```python
from build123d import *

# Parameters (mm, degrees)
SKETCH1_R           = 44.45
BOSS_EXTRUDE1_DEPTH = 1000


with BuildPart() as part:
    # Sketch1 → Boss-Extrude1 (new body)
    with BuildSketch(Plane(origin=(0, 0, 0), x_dir=(1, 0, 0), z_dir=(0, 1, 0))):
        with Locations(Location((0, 0, 0), (0, 0, 270))):
            Circle(SKETCH1_R)
    extrude(amount=BOSS_EXTRUDE1_DEPTH)

    # Sketch3 → Revolve3 (revolve)
    with BuildSketch(Plane.XY, mode=Mode.PRIVATE) as revolve3_sk:
        Polygon((0, 1000), (0, 1276.86), (-44.45, 1000), align=None)
    revolve(revolve3_sk.sketch.rotate(Axis((0, 1000, 0), (0, 1, 0)), 270), axis=Axis((0, 1000, 0), (0, 1, 0)))

    # Sketch4 → Revolve4 (revolve)
    with BuildSketch(Plane.XY):
        Polygon((0, 0), (0, -276.86), (-44.45, 0), align=None)
    revolve(axis=Axis((0, 0, 0), (0, -1, 0)))


solid = part.part
```
Here's how the part is built. I have some questions about the finished solid (model axes, mm). Coordinates: 2 decimals unless noted, no trailing zeros. Write each loop counter-clockwise with the first axis right and the second up, starting at its lowest first coordinate (ties: lowest second). Pieces come first, ordered by that corner, then holes. Notation, with made-up numbers: M 2.25,67 L 21.25,67 A24 cw 21.25,81 Z; hole C 73.25,-1 d1. An arc over 180 degrees is marked long. Answer as CSV lines item,"result". Start each with the question number.
Q1. Will these pins go through, and if not, where does the flat tip stop? pin 1 Ø1 at (y, z) = (57.5, -31.5) entering from -X; pin 2 Ø6 at (x, y) = (-3, 753.5) entering from -Z; pin 3 Ø1 at (y, z) = (978.5, 9) entering from -X; pin 4 Ø3 at (x, y) = (-5.5, 353.5) entering from +Z.
Q2. I need wall thicknesses on probe 1 along X at (y, z) = (796, -0.5); probe 2 along Z at (x, y) = (-22, 754); probe 3 along Z at (x, y) = (25, -33). Which ranges of each line are inside material? Lowest first, please. Write a range as [from, to].
Q3. Suppose I cut it at B-B, the plane y = -157. List the corners of the cut face in (x, z) for me, then the cut area to 3 significant figures.
Q4. Suppose I cut it at A-A, the plane y = 699. List the corners of the cut face in (x, z) for me, then the cut area to 3 significant figures.
Entries:
1,pin 1,"stops at x = -31.86"
1,pin 2,"stops at z = -44.45"
1,pin 3,"stops at x = -43.63"
1,pin 4,"stops at z = 44.27"
2,probe 1,"x = [-44.45, 44.45]"
2,probe 2,"z = [-38.62, 38.62]"
2,probe 3,"z = [-30.13, 30.13]"
3,outline,"C 0,0 d38.49"
3,area,"1,160 mm²"
4,outline,"C 0,0 d88.9"
4,area,"6,210 mm²"
